Geometry: final body of the model. Coordinates: model frame, mm. A direction names the side the tool comes from. Give positions to 0.01 mm unless a question says otherwise; leave off trailing zeros. Loops run counter-clockwise (first coordinate to the right, second up) from the corner with the lowest first, then second, coordinate; pieces in that order, holes last.
1. Section B-B, the plane z = -0.5. Output: boundary loops of the cut face in (x, y).
2. First-contact query: P1, Ø0.9, axis at y = 8.5, z = 2.5, coming from the +X side; P2, Ø2, axis at x = 5.5, y = -5.5, coming from the +Z side; P3, Ø3, axis at x = -2.5, z = -0.5, coming from the -Y side. Flat tips, straight axial feed; report the tip coordinate or a pass-through.
3. Section A-A, the plane y = -4.5. Output: boundary loops of the cut face in (x, z), then the cut area to 3 significant figures.
4. Material intervals for line 1 along Z through (x, y) = (-3.5, 6.5); line 2 along Y through (x, z) = (-0.5, 0.25); line 3 along X through (y, z) = (3.25, -4), sorted ascending.
5. Section D-D, the plane y = 6.5. State how many separate pieces and enclosed holes the cut face has, then the cut area to 3 significant figures.
6. Draft query along X for faces 4 (the face through (5.9, -0.07, 0.79)), 5 (the face through (1.416, 6.448, -3.099)), 6 (the face through (-2, 0, -4.685)). Return one class per face: +X half, -X half, draft (parallel to the pull), parting line (faces both ways), or undercut.
7. Access query for faces 1 (the face through (0, 10, -3)), 2 (the face through (0, 10, 3)), 3 (the face through (1.26, 0.07, -0.79)). Directions: +Z, -Z, +X, -X, +Y, -Y. A direction counts if a zero-diameter tool reaches every point of the face in a straight line with its end or side. Return the directions, or none.
8. Section C-C, the plane z = -3.75. Output: boundary loops of the cut face in (x, y).
from build123d import *

# Parameters (mm, degrees)
F4_ANGLE       = 90
F6_ANGLE       = 90
F7_DEPTH       = 10
F10_DEPTH      = 3.1295758847
F11_DEPTH      = 3.1295758847
F13_DEPTH      = 14.5
F13_DEPTH_BACK = 25


with BuildPart() as f4:
    # F3 (on plane+point) → F4 (revolve)
    with BuildSketch(Plane.XZ.offset(-5.0000661737)):
        Polygon((-2.8551849101, 2.3852105297), (-2.0256090254, 1.555634645), (-0.4699743804, 0), (-2.0256090254, -1.555634645), (0, -1.555634645), (0, 0), (0, 1.555634645), (0, 4.6852105297), (-7.1624873409, 4.6852105297), (-7.1624873409, 1.555634645), (-7.1624873409, -1.555634645), (-5.1368783154, -1.555634645), (-6.6925129605, 0), (-5.1368783154, 1.555634645), (-4.3073024307, 2.3852105297), (-3.5812436704, 3.11126929), align=None)
        Polygon((-4.3073024307, -2.3852105297), (-5.1368783154, -1.555634645), (-7.1624873409, -1.555634645), (-7.1624873409, -4.6852105297), (0, -4.6852105297), (0, -1.555634645), (-2.0256090254, -1.555634645), (-2.8551849101, -2.3852105297), (-3.5812436704, -3.11126929), align=None)
        Polygon((-2.8551849101, -2.3852105297), (-3.5812436704, -2.3852105297), (-3.5812436704, -3.11126929), align=None)
        Polygon((-3.5812436704, -3.11126929), (-3.5812436704, -2.3852105297), (-4.3073024307, -2.3852105297), align=None)
    revolve(axis=Axis((0, 5.0000661737, -0.016850885), (0, 0, -1)), revolution_arc=F4_ANGLE)

    # F5 (on face) → F6 (revolve)
    with BuildSketch(Plane.YZ):
        Polygon((5.4700405542, 0), (7.0256751992, 1.555634645), (5.0000661737, 1.555634645), (5.0000661737, -1.555634645), (7.0256751992, -1.555634645), align=None)
        Polygon((12.1625535146, 1.555634645), (10.1369444892, 1.555634645), (11.6925791342, 0), (10.1369444892, -1.555634645), (12.1625535146, -1.555634645), align=None)
    revolve(axis=Axis((0, 5.0000661737, -0.016850885), (0, 0, -1)), revolution_arc=F6_ANGLE)

    # F7 (add): faces of the model
    f7_faces = [f4.faces().sort_by_distance(p)[0] for p in [
        (7.1253617587, 5.0000661737, 0),
        (-1.9422105795, 5.0000661737, 1.639033091),
        (1.0128045127, 5.0000661737, -1.5185090628),
    ]]
    extrude(f7_faces, amount=F7_DEPTH)

    # F8: F4 across plane


with BuildPart() as f4_1:
    add(f4.part)
    add(f4.part.mirror(Plane.XZ))

    # F9: F4 across plane


with BuildPart() as f4_2:
    add(f4_1.part)
    add(f4_1.part.mirror(Plane.XY))

    # F10 (add, through all): faces of the model
    f10_faces = [f4_2.faces().sort_by_distance(p)[0] for p in [
        (0.8596951711, 5.8597613449, -1.555634645),
        (1.0128045127, 5, -1.555634645),
        (1.0128045127, 0, -1.555634645),
        (1.0128045127, -5, -1.555634645),
        (0.8596951711, -5.8597613449, -1.555634645),
    ]]
    extrude(f10_faces, amount=F10_DEPTH)

    # F11 (add, through all): faces of the model
    f11_faces = [f4_2.faces().sort_by_distance(p)[0] for p in [
        (0.8596951711, 5.8597613449, 1.555634645),
        (1.0128045127, 5, 1.555634645),
        (1.0128045127, 0, 1.555634645),
        (1.0128045127, -5, 1.555634645),
        (0.8596951711, -5.8597613449, 1.555634645),
    ]]
    extrude(f11_faces, amount=F11_DEPTH)

    # F12 (on Front) → F13 (cut, two sides)
    with BuildSketch(Plane.XZ) as f13_sk:
        Polygon((-5.1368783154, -6.1799879186), (-5.1368783154, 5.2285962738), (-8.7532252073, 5.3635202348), (-9.4878124073, -3.8263113238), align=None)
    extrude(amount=-F13_DEPTH, mode=Mode.SUBTRACT)
    extrude(f13_sk.sketch, amount=F13_DEPTH_BACK, mode=Mode.SUBTRACT)


solid = f4_2.part
Answers below:
1. outline: (-5.14, -9.99) arc R7.16 ccw to (7.16, -5) - (7.16, 5) arc R7.16 ccw to (-5.14, 9.99) - (-5.14, 8.46) arc R6.19 cw to (6.19, 5) - (6.19, -5) arc R6.19 cw to (-5.14, -8.46) - close; (-0.97, -5) arc R0.97 ccw to (0.97, -5) - (0.97, 5) arc R0.97 ccw to (-0.97, 5) - close
2. P1: stops at x = 0
2. P2: stops at z = 1.56
2. P3: stops at y = -12.09
3. outline: (-5.14, -4.69) - (2.03, -4.69) - (2.03, -1.56) - (0.47, 0) - (2.03, 1.56) - (2.03, 4.69) - (-5.14, 4.69) - (-5.14, 1.56) - (-4.31, 2.39) - (-2.86, 2.39) - (-0.47, 0) - (-2.86, -2.39) - (-4.31, -2.39) - (-5.14, -1.56) - close; (5.14, -1.56) - (7.16, -1.56) - (7.16, 1.56) - (5.14, 1.56) - (6.69, 0) - close
3. area: 52.7 mm2
4. line 1: z = -4.69 to -2.39, 2.39 to 4.69
4. line 2: y = -12.15 to -11.42, -5.52 to 5.52, 11.42 to 12.15
4. line 3: x = -5.14 to 2.03
5. separate pieces: 3
5. enclosed holes: 0
5. area: 42.3 mm2
6. face 4: undercut
6. face 5: +X half
6. face 6: draft
7. face 1: -Z, +X, +Y
7. face 2: +Z, +X, +Y
7. face 3: none
8. outline: (-5.14, -9.99) arc R7.16 ccw to (0, -12.16) - (0, -7.03) arc R2.03 ccw to (2.03, -5) - (2.03, 5) arc R2.03 ccw to (0, 7.03) - (0, 12.16) arc R7.16 ccw to (-5.14, 9.99) - close
